Could you check a few things on this model? Use its own coordinates, in mm. Face numbers are marked on the shaded views. A direction names the side the tool comes from. Give positions to 0.01 mm unless a question says otherwise; leave off trailing zeros. Order: outer loops, then holes, each group sorted by start corner. A loop starts at its lowest first (then second) coordinate and runs counter-clockwise, first axis right, second up. Notation, with made-up numbers: M 73,39 L 86,39 A33 cw 86,67 Z; hole C -20.75,20 d2. An arc over 180 degrees is marked long. Use a Markdown table: item, result. Add a question column.
Item 1: For the marked faces 4 and 5, which set-ups out of +Z, -Z, +X, -X, +Y, -Y let a thin tool reach every point of the face, with its end or its side?
Item 2: Suppose I cut it at C-C on x = 7. Write out the boundary of the cut face in (y, z), plus the area to 3 significant figures.
Item 3: Suppose I cut it at D-D on y = -18.5. Write out the boundary of the cut face in (x, z), plus the area to 3 significant figures.
Item 4: Suppose I cut it at A-A on x = 0. Write out the boundary of the cut face in (y, z), plus the area to 3 significant figures.
Item 5: I'm going to push flat-ended pins straight in: pin 1 Ø10.5 at (x, y) = (10, -11) entering from +Z; pin 2 Ø0.8 at (y, z) = (24.5, 9) entering from +X; pin 3 Ø0.8 at (x, y) = (11.5, 24.5) entering from +Z. Where does each tip first touch, or does it pass through?
Item 6: If we mould it in two halves opening along X, with no side actions, what happens to the marked faces 1, 2 and 3? For each: released by +X, released by -X, zero draft, split by the parting line, or undercut.
Item 7: Suppose I cut it at B-B on y = 5. Write out the boundary of the cut face in (x, z).
Item 8: If I drill on L1, parallel to X at y = 14.5, z = 2; L2, parallel to X at y = 6.5, z = 4; L3, parallel to Y at x = 7.5, z = 2, over which ranges is the centre line in solid material (lowest first)? Write a range as from..to.
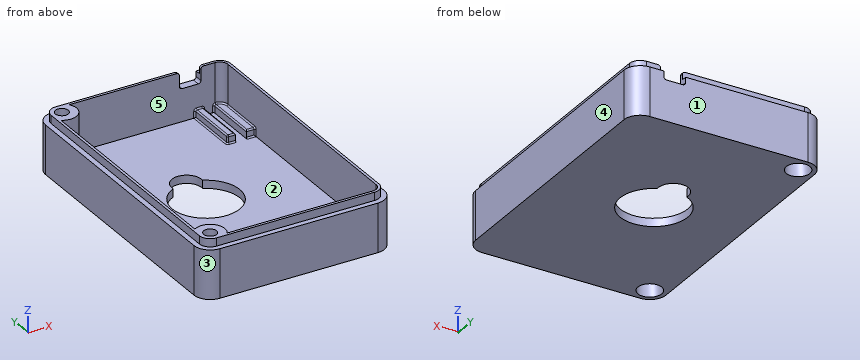
from build123d import *

# Parameters (mm, degrees)
EXRUDE_BASE_DEPTH       = 1.5
EXTRUDE_SIDEWALLS_DEPTH = 9
PARTLING_LINE_LIP_START = -1.5
PARTLING_LINE_LIP_DEPTH = 1.5
SKETCH4_W               = 1.5
SKETCH4_H               = 10
SKETCH4_W_2             = 2.151899305
BOSS_EXTRUDE3_DEPTH     = 1.5
FILLET2_R               = 0.25
CUT_EXTRUDE2_DEPTH      = 1.5
FILLET3_R               = 0.5
SCREWBOSS_DEPTH         = 9
SCREWHOLE_DEPTH         = 34.88613029
SCREWHOLE_DEPTH_BACK    = 34.88613029
SCREW_HOLES_R           = 1.2
SKETCH8_R               = 2.2
CUT_EXTRUDE4_DEPTH      = 2.6


with BuildPart() as part:
    # Sketch1 → Exrude-Base (new body)
    with BuildSketch(Plane.XY):
        with BuildLine():
            Line((9.739580757, 25.295602697), (12.739580757, 25.295602697))
            Line((12.739580757, 25.295602697), (13.239580757, 25.295602697))
            Line((13.239580757, 25.295602697), (13.739580757, 25.295602697))
            Line((13.739580757, 25.295602697), (15.834580757, 25.295602697))
            ThreePointArc((15.834580757, 25.295602697), (17.9559011, 24.41692304), (18.834580757, 22.295602697))
            Line((18.834580757, 22.295602697), (18.834580757, -23.693227454))
            ThreePointArc((18.834580757, -23.693227454), (17.9559011, -25.814547798), (15.834580757, -26.693227454))
            Line((15.834580757, -26.693227454), (-13.365419243, -26.693227454))
            ThreePointArc((-13.365419243, -26.693227454), (-15.486739587, -25.814547798), (-16.365419243, -23.693227454))
            Line((-16.365419243, -23.693227454), (-16.365419243, 22.295602697))
            ThreePointArc((-16.365419243, 22.295602697), (-15.486739587, 24.41692304), (-13.365419243, 25.295602697))
            Line((-13.365419243, 25.295602697), (8.739580757, 25.295602697))
            Line((8.739580757, 25.295602697), (9.239580757, 25.295602697))
            Line((9.239580757, 25.295602697), (9.739580757, 25.295602697))
        make_face()
        with BuildLine():
            ThreePointArc((-2.72431184, 5.625), (0, -6.25), (2.72431184, 5.625))
            ThreePointArc((2.72431184, 5.625), (0, 8.75), (-2.72431184, 5.625))
        make_face(mode=Mode.SUBTRACT)
    extrude(amount=EXRUDE_BASE_DEPTH)

    # Sketch2 → Extrude-Sidewalls (add)
    with BuildSketch(Plane.XY.offset(1.5)):
        with BuildLine():
            Line((18.834580757, 22.295602697), (18.834580757, -23.693227454))
            ThreePointArc((18.834580757, -23.693227454), (17.9559011, -25.814547798), (15.834580757, -26.693227454))
            Line((15.834580757, -26.693227454), (-13.365419243, -26.693227454))
            ThreePointArc((-13.365419243, -26.693227454), (-15.486739587, -25.814547798), (-16.365419243, -23.693227454))
            Line((-16.365419243, -23.693227454), (-16.365419243, 22.295602697))
            ThreePointArc((-16.365419243, 22.295602697), (-15.486739587, 24.41692304), (-13.365419243, 25.295602697))
            Line((-13.365419243, 25.295602697), (15.834580757, 25.295602697))
            ThreePointArc((15.834580757, 25.295602697), (17.9559011, 24.41692304), (18.834580757, 22.295602697))
        make_face()
        with BuildLine():
            Line((17.334580757, 22.295602697), (17.334580757, -23.693227454))
            ThreePointArc((17.334580757, -23.693227454), (16.895240929, -24.753887626), (15.834580757, -25.193227454))
            Line((15.834580757, -25.193227454), (-13.365419243, -25.193227454))
            ThreePointArc((-13.365419243, -25.193227454), (-14.426079415, -24.753887626), (-14.865419243, -23.693227454))
            Line((-14.865419243, -23.693227454), (-14.865419243, 22.295602697))
            ThreePointArc((-14.865419243, 22.295602697), (-14.426079415, 23.356262868), (-13.365419243, 23.795602697))
            Line((-13.365419243, 23.795602697), (15.834580757, 23.795602697))
            ThreePointArc((15.834580757, 23.795602697), (16.895240929, 23.356262868), (17.334580757, 22.295602697))
        make_face(mode=Mode.SUBTRACT)
    extrude(amount=EXTRUDE_SIDEWALLS_DEPTH)

    # Sketch3 → Partling-Line-Lip (cut)
    with BuildSketch(Plane.XY.offset(10.5).offset(PARTLING_LINE_LIP_START)):
        with BuildLine():
            Line((18.834580757, 22.295602697), (18.834580757, -23.693227454))
            ThreePointArc((18.834580757, -23.693227454), (17.9559011, -25.814547798), (15.834580757, -26.693227454))
            Line((15.834580757, -26.693227454), (-13.365419243, -26.693227454))
            ThreePointArc((-13.365419243, -26.693227454), (-15.486739587, -25.814547798), (-16.365419243, -23.693227454))
            Line((-16.365419243, -23.693227454), (-16.365419243, 22.295602697))
            ThreePointArc((-16.365419243, 22.295602697), (-15.486739587, 24.41692304), (-13.365419243, 25.295602697))
            Line((-13.365419243, 25.295602697), (15.834580757, 25.295602697))
            ThreePointArc((15.834580757, 25.295602697), (17.9559011, 24.41692304), (18.834580757, 22.295602697))
        make_face()
        with BuildLine():
            Line((17.834580757, 22.295602697), (17.834580757, -23.693227454))
            ThreePointArc((17.834580757, -23.693227454), (17.248794319, -25.107441017), (15.834580757, -25.693227454))
            Line((15.834580757, -25.693227454), (-13.365419243, -25.693227454))
            ThreePointArc((-13.365419243, -25.693227454), (-14.779632806, -25.107441017), (-15.365419243, -23.693227454))
            Line((-15.365419243, -23.693227454), (-15.365419243, 22.295602697))
            ThreePointArc((-15.365419243, 22.295602697), (-14.779632806, 23.709816259), (-13.365419243, 24.295602697))
            Line((-13.365419243, 24.295602697), (15.834580757, 24.295602697))
            ThreePointArc((15.834580757, 24.295602697), (17.248794319, 23.709816259), (17.834580757, 22.295602697))
        make_face(mode=Mode.SUBTRACT)
    extrude(amount=PARTLING_LINE_LIP_DEPTH, mode=Mode.SUBTRACT)

    # Sketch4 → Boss-Extrude3 (add)
    with BuildSketch(Plane.XY.offset(1.5)):
        with Locations((12.909580757, 18.795602697)):
            Rectangle(SKETCH4_W, SKETCH4_H)
        with Locations((16.73553041, 18.795602697)):
            Rectangle(SKETCH4_W_2, SKETCH4_H)
    extrude(amount=BOSS_EXTRUDE3_DEPTH)

    # Fillet2
    fillet2_edges = [part.edges().sort_by_distance(p)[0] for p in [
        (13.659580757, 18.795602697, 3),
        (12.159580757, 18.795602697, 3),
        (12.159580757, 13.795602697, 2.25),
        (16.497080757, 13.795602697, 3),
        (15.659580757, 18.795602697, 3),
        (12.909580757, 13.795602697, 3),
    ]]
    fillet(fillet2_edges, radius=FILLET2_R)
    fillet2_2_edges = [part.edges().sort_by_distance(p)[0] for p in [
        (13.659580757, 23.795602697, 2.125),
        (13.034580757, 13.795602697, 1.5),
        (17.334580757, 13.795602697, 2.125),
        (15.659580757, 23.795602697, 2.125),
        (12.909580757, 23.795602697, 3),
        (12.159580757, 23.795602697, 2.125),
        (12.159580757, 18.920602697, 1.5),
        (17.334580757, 18.170602697, 3),
        (16.921434013, 23.329406353, 3),
        (16.497080757, 13.795602697, 1.5),
        (15.871629396, 23.795145092, 2.997102598),
        (15.708024313, 23.795602697, 2.897901995),
        (17.334580757, 13.868826001, 2.926776695),
        (12.232804061, 13.868826001, 1.5),
        (12.232804061, 23.795602697, 2.926776695),
        (13.586357452, 23.795602697, 2.926776695),
    ]]
    fillet(fillet2_2_edges, radius=FILLET2_R)

    # Sketch5 → Cut-Extrude2 (cut)
    with BuildSketch(Plane(origin=(0, 25.295602697, 0), x_dir=(1, 0, 0), z_dir=(0, 1, 0))):
        with BuildLine():
            Line((9.239580757, -10.5), (9.239580757, -8))
            ThreePointArc((9.239580757, -8), (9.386027366, -7.646446609), (9.739580757, -7.5))
            Line((9.739580757, -7.5), (12.739580757, -7.5))
            ThreePointArc((12.739580757, -7.5), (13.093134147, -7.646446609), (13.239580757, -8))
            Line((13.239580757, -8), (13.239580757, -10.5))
            Line((13.239580757, -10.5), (9.239580757, -10.5))
        make_face()
    extrude(amount=-CUT_EXTRUDE2_DEPTH, mode=Mode.SUBTRACT)

    # Fillet3
    fillet3_edges = [part.edges().sort_by_distance(p)[0] for p in [
        (13.239580757, 24.045602697, 10.5),
        (9.239580757, 24.045602697, 10.5),
    ]]
    fillet(fillet3_edges, radius=FILLET3_R)

    # Sketch7 → ScrewBoss (add)
    with BuildSketch(Plane.XY.offset(1.5)):
        with BuildLine():
            Line((-13.365419243, -25.193227454), (-11.120424811, -25.193227454))
            ThreePointArc((-11.120424811, -25.193227454), (-11.456230934, -21.784039145), (-14.865419243, -21.448233022))
            Line((-14.865419243, -21.448233022), (-14.865419243, -23.693227454))
            ThreePointArc((-14.865419243, -23.693227454), (-14.426079415, -24.753887626), (-13.365419243, -25.193227454))
        make_face()
        with BuildLine():
            Line((-11.120424811, 23.795602697), (-13.365419243, 23.795602697))
            ThreePointArc((-13.365419243, 23.795602697), (-14.426079415, 23.356262868), (-14.865419243, 22.295602697))
            Line((-14.865419243, 22.295602697), (-14.865419243, 20.050608265))
            ThreePointArc((-14.865419243, 20.050608265), (-11.456230934, 20.386414387), (-11.120424811, 23.795602697))
        make_face()
    extrude(amount=SCREWBOSS_DEPTH)

    # Screw-Holes → ScrewHole (cut, two sides: drawn at the far end of the back side and taken through both)
    with BuildSketch(Plane.XY.offset(1.5).offset(-SCREWHOLE_DEPTH_BACK)):
        with Locations((-13.365419243, 22.295602697)):
            Circle(SCREW_HOLES_R)
        with Locations((-13.365419243, -23.693227454)):
            Circle(SCREW_HOLES_R)
    extrude(amount=SCREWHOLE_DEPTH + SCREWHOLE_DEPTH_BACK, mode=Mode.SUBTRACT)

    # Sketch8 → Cut-Extrude4 (cut)
    with BuildSketch(Plane(origin=(0, 0, 0), x_dir=(-1, 0, 0), z_dir=(0, 0, -1))):
        with Locations((13.365419243, 22.295602697)):
            Circle(SKETCH8_R)
        with Locations((13.365419243, -23.693227454)):
            Circle(SKETCH8_R)
    extrude(amount=-CUT_EXTRUDE4_DEPTH, mode=Mode.SUBTRACT)


solid = part.part
Findings below:
| question | item | result |
|---|---|---|
| 1 | face 4 | +Z, -Z, +X, +Y, -Y |
| 1 | face 5 | +Z |
| 2 | outline | M -26.69,0 L 25.3,0 L 25.3,9 L 24.3,9 L 24.3,10.5 L 23.8,10.5 L 23.8,1.5 L -25.19,1.5 L -25.19,10.5 L -25.69,10.5 L -25.69,9 L -26.69,9 Z |
| 2 | area | 102 mm^2 |
| 3 | outline | M -16.37,0 L 18.83,0 L 18.83,9 L 17.83,9 L 17.83,10.5 L 17.33,10.5 L 17.33,1.5 L -14.87,1.5 L -14.87,10.5 L -15.37,10.5 L -15.37,9 L -16.37,9 Z |
| 3 | area | 76.8 mm^2 |
| 4 | outline | M -26.69,0 L -6.25,0 L -6.25,1.5 L -25.19,1.5 L -25.19,10.5 L -25.69,10.5 L -25.69,9 L -26.69,9 Z; M 8.75,0 L 25.3,0 L 25.3,9 L 24.3,9 L 24.3,10.5 L 23.8,10.5 L 23.8,1.5 L 8.75,1.5 Z |
| 4 | area | 79.5 mm^2 |
| 5 | pin 1 | stops at z = 1.5 |
| 5 | pin 2 | stops at x = 18.23 |
| 5 | pin 3 | stops at z = 7.5 |
| 6 | face 1 | zero draft |
| 6 | face 2 | undercut |
| 6 | face 3 | released by -X |
| 7 | outline | M -16.37,0 L -3.75,0 L -3.75,1.5 L -14.87,1.5 L -14.87,10.5 L -15.37,10.5 L -15.37,9 L -16.37,9 Z; M 3.75,0 L 18.83,0 L 18.83,9 L 17.83,9 L 17.83,10.5 L 17.33,10.5 L 17.33,1.5 L 3.75,1.5 Z |
| 8 | L1 | x = -16.37..-14.87, 12.16..13.66, 15.66..18.83 |
| 8 | L2 | x = -16.37..-14.87, 17.33..18.83 |
| 8 | L3 | y = -26.69..-25.19, 23.8..25.3 |
